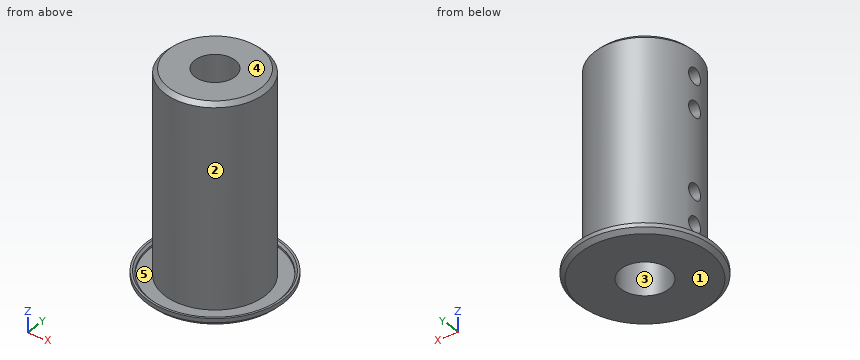
```python
from build123d import *

# Parameters (mm, degrees)
F0_R     = 12.5
F0_R_2   = 6
F0_R_3   = 5
F1_DEPTH = 25
F2_DEPTH = 25
F3_R     = 2
F4_DEPTH = 25
F5_SIZE  = 1
F6_R     = 17
F6_R_2   = 16
F6_R_3   = 12.5
F6_R_4   = 6
F7_DEPTH = 1
F8_DEPTH = 1
F9_SIZE  = 0.5
F10_SIZE = 0.99999


# Not quite as in the source:
# - a fillet or chamfer is up to 0.001 mm smaller than in the source, because OpenCascade refuses the exact size


with BuildPart() as f1:
    # F0 (on Top) → F1 (new body)
    with BuildSketch(Plane.XY):
        Circle(F0_R)
        Circle(F0_R_2, mode=Mode.SUBTRACT)
        Circle(F0_R_2)
        Circle(F0_R_3, mode=Mode.SUBTRACT)
    extrude(amount=F1_DEPTH)

    # F0 (on Top) → F2 (join)
    with BuildSketch(Plane.XY):
        Circle(F0_R)
        Circle(F0_R_2, mode=Mode.SUBTRACT)
    extrude(amount=-F2_DEPTH)

    # F3 (on Right) → F4 (cut)
    with BuildSketch(Plane.YZ):
        with Locations((0, -18)):
            Circle(F3_R)
        with Locations((0, -10)):
            Circle(F3_R)
        with Locations((0, 10)):
            Circle(F3_R)
        with Locations((0, 18)):
            Circle(F3_R)
    extrude(amount=-F4_DEPTH, mode=Mode.SUBTRACT)

    # F5
    f5_edges = [f1.edges().sort_by_distance(p)[0] for p in [
        (-12.5, 0, 25),
    ]]
    chamfer(f5_edges, length=F5_SIZE)

    # F6 (on face) → F7 (join)
    with BuildSketch(Plane(origin=(0, 0, -25), x_dir=(1, 0, 0), z_dir=(0, 0, -1))):
        Circle(F6_R)
        Circle(F6_R_2, mode=Mode.SUBTRACT)
        Circle(F6_R_2)
        Circle(F6_R_3, mode=Mode.SUBTRACT)
        Circle(F6_R_3)
        Circle(F6_R_4, mode=Mode.SUBTRACT)
    extrude(amount=F7_DEPTH)

    # F6 (on face) → F8 (join)
    with BuildSketch(Plane(origin=(0, 0, -25), x_dir=(1, 0, 0), z_dir=(0, 0, -1))):
        Circle(F6_R)
        Circle(F6_R_2, mode=Mode.SUBTRACT)
    extrude(amount=-F8_DEPTH)

    # F9
    f9_edges = [f1.edges().sort_by_distance(p)[0] for p in [
        (-16, 0, -24),
    ]]
    chamfer(f9_edges, length=F9_SIZE)

    # F10 (size 1 in the source; OpenCascade refuses exactly that, so slightly less here)
    f10_edges = [f1.edges().sort_by_distance(p)[0] for p in [
        (-17, 0, -26),
    ]]
    chamfer(f10_edges, length=F10_SIZE)


solid = f1.part
```
Check sheet for the modelled part. Datum: model origin and axes. Units: mm. Face numbers are marked on the shaded views. A direction names the side the tool comes from. Give positions to 0.01 mm unless a question says otherwise; leave off trailing zeros. Order: outer loops, then holes, each group sorted by start corner. A loop starts at its lowest first (then second) coordinate and runs counter-clockwise, first axis right, second up. Notation, with made-up numbers: M 34.25,-23 L 70.25,-23 A19 ccw 70.25,-16 Z; hole C -23,12 d9. An arc over 180 degrees is marked long. Answer in a Markdown table with one row per item.
1) Gauge pin test, flat ends, axial feed: P1, Ø3.5, axis at x = -1, y = 1.5, coming from the -Z side; P2, Ø6.5, axis at y = 0, z = 10, coming from the -X side; P3, Ø3, axis at y = -10.5, z = 16.5, coming from the +X side; P4, Ø1, axis at x = -3, z = 20, coming from the -Y side. Record the tip position at first contact, or that the pin passes through.
Filled sheet:
| item | result |
|---|---|
| P1 | passes through |
| P2 | stops at x = -12.5 |
| P3 | stops at x = 8.67 |
| P4 | stops at y = -12.25 |
2) Access from +Z, -Z, +X, -X, +Y, -Y to the whole of each face (thin tool, end or side, straight path). Record for the marked faces 1 and 2.
Filled sheet:
| item | result |
|---|---|
| face 1 | -Z, +X, -X, +Y, -Y |
| face 2 | +Z |
3) Cross-section at A-A, the plane x = 0. Enter the section's corners in (y, z), plus the area to 3 significant figures.
Filled sheet:
| item | result |
|---|---|
| outline | M -17,-25 L -16,-26 L -6,-26 L -6,0 L -5,0 L -5,25 L -11.5,25 L -12.5,24 L -12.5,-25 L -16,-25 L -16,-24.5 L -16.5,-24 L -17,-24 Z; M 5,0 L 6,0 L 6,-26 L 16,-26 L 17,-25 L 17,-24 L 16.5,-24 L 16,-24.5 L 16,-25 L 12.5,-25 L 12.5,24 L 11.5,25 L 5,25 Z |
| area | 722 mm2 |
4) Cross-section at C-C, the plane z = 6. Enter the section's corners in (x, y).
Filled sheet:
| item | result |
|---|---|
| outline | C 0,0 d25; hole C 0,0 d10 |
5) Release check for a two-part mould opening along Y. For the marked faces 3, 4 and 5 record: +Y half, -Y half, draft (parallel to the pull), parting line (faces both ways), or undercut.
Filled sheet:
| item | result |
|---|---|
| face 3 | undercut |
| face 4 | draft |
| face 5 | undercut |
6) Thickness scan on L1, parallel to Y at x = 0, z = -19.25; L2, parallel to Y at x = -4.5, z = -5; L3, parallel to Z at x = -9, y = -10.5. Record the ranges inside material, lowest first. Write a range as [from, to].
Filled sheet:
| item | result |
|---|---|
| L1 | y = [-12.5, -6], [6, 12.5] |
| L2 | y = [-11.66, -3.97], [3.97, 11.66] |
| L3 | z = [-26, -25] |
7) Cross-section at B-B, the plane y = 0. Count the separate pieces of the cut face and the enclosed holes in it, plus the area to 3 significant figures.
Filled sheet:
| item | result |
|---|---|
| separate pieces | 6 |
| enclosed holes | 0 |
| area | 610 mm2 |
